```python
from build123d import *

# Parameters (mm, degrees)
SHELL1_T            = -1
LPATTERN1_COUNT     = 8
LPATTERN1_PITCH     = 9
SKETCH3_W           = 8
SKETCH3_H           = 92.26
BOSS_EXTRUDE1_DEPTH = 1
CHAMFER1_SIZE       = 1
SKETCH4_R           = 2.5
CUT_EXTRUDE1_DEPTH  = 82.991962069
CHAMFER2_SIZE       = 1
SKETCH5_W           = 3
SKETCH5_H           = 2
CUT_EXTRUDE2_DEPTH  = 84.346756649
LPATTERN2_COUNT     = 8
LPATTERN2_PITCH     = 9


with BuildPart() as part:
    # Sketch1 → Revolve1 (revolve)
    with BuildSketch(Plane.XY, mode=Mode.PRIVATE) as revolve1_sk:
        Polygon((0, 30), (3, 30), (3, 0), (2.1, -5), (0, -5), align=None)
    revolve(revolve1_sk.sketch.rotate(Axis((0, 30, 0), (0, -1, 0)), 180), axis=Axis((0, 30, 0), (0, -1, 0)))

    # Shell1
    shell1_openings = [part.faces().sort_by_distance(p)[0] for p in [
        (0, -5, 0),
        (0, 30, 0),
    ]]
    offset(amount=SHELL1_T, openings=shell1_openings, kind=Kind.INTERSECTION)


with BuildPart() as lpattern1_1:
    # LPattern1: pattern copy
    add(part.part.moved(Location(Vector(0, 0, 1) * (1 * LPATTERN1_PITCH))))


with BuildPart() as lpattern1_2:
    # LPattern1: pattern copy
    add(part.part.moved(Location(Vector(0, 0, 1) * (2 * LPATTERN1_PITCH))))


with BuildPart() as lpattern1_3:
    # LPattern1: pattern copy
    add(part.part.moved(Location(Vector(0, 0, 1) * (3 * LPATTERN1_PITCH))))


with BuildPart() as lpattern1_4:
    # LPattern1: pattern copy
    add(part.part.moved(Location(Vector(0, 0, 1) * (4 * LPATTERN1_PITCH))))


with BuildPart() as lpattern1_5:
    # LPattern1: pattern copy
    add(part.part.moved(Location(Vector(0, 0, 1) * (5 * LPATTERN1_PITCH))))


with BuildPart() as lpattern1_6:
    # LPattern1: pattern copy
    add(part.part.moved(Location(Vector(0, 0, 1) * (6 * LPATTERN1_PITCH))))


with BuildPart() as lpattern1_7:
    # LPattern1: pattern copy
    add(part.part.moved(Location(Vector(0, 0, 1) * (7 * LPATTERN1_PITCH))))


with BuildPart() as part_1:
    add(part.part)

    add(lpattern1_1.part)  # Boss-Extrude1 merges LPattern1_1

    add(lpattern1_2.part)  # Boss-Extrude1 merges LPattern1_2

    add(lpattern1_3.part)  # Boss-Extrude1 merges LPattern1_3

    add(lpattern1_4.part)  # Boss-Extrude1 merges LPattern1_4

    add(lpattern1_5.part)  # Boss-Extrude1 merges LPattern1_5

    add(lpattern1_6.part)  # Boss-Extrude1 merges LPattern1_6

    add(lpattern1_7.part)  # Boss-Extrude1 merges LPattern1_7
    # Sketch3 → Boss-Extrude1 (add, symmetric)
    with BuildSketch(Plane(origin=(0, 3, 0), x_dir=(-1, 0, 0), z_dir=(0, -1, 0))):
        with Locations((0, -31.527464831)):
            Rectangle(SKETCH3_W, SKETCH3_H)
    extrude(amount=BOSS_EXTRUDE1_DEPTH, both=True)

    # Chamfer1
    chamfer1_edges = [part_1.edges().sort_by_distance(p)[0] for p in [
        (3, 4, 0),
        (3, 2, 0),
        (3, 4, 9),
        (3, 2, 9),
        (3, 4, 18),
        (3, 2, 18),
        (3, 4, 27),
        (3, 2, 27),
        (3, 4, 36),
        (3, 2, 36),
        (3, 4, 45),
        (3, 2, 45),
        (3, 4, 54),
        (3, 2, 54),
        (3, 4, 63),
        (3, 2, 63),
    ]]
    chamfer(chamfer1_edges, length=CHAMFER1_SIZE - 0.0001)  # a hair under: the kernel refuses the full size

    # Sketch4 → Cut-Extrude1 (cut, through all)
    with BuildSketch(Plane(origin=(0, 4, 0), x_dir=(1, 0, 0), z_dir=(0, 1, 0))):
        with Locations(Location((0, -73.63, 0), (0, 0, 270))):
            Circle(SKETCH4_R)
        with Locations(Location((0, 10.63, 0), (0, 0, 270))):
            Circle(SKETCH4_R)
    extrude(amount=-CUT_EXTRUDE1_DEPTH, mode=Mode.SUBTRACT)

    # Chamfer2
    chamfer2_edges = [part_1.edges().sort_by_distance(p)[0] for p in [
        (0, 2, 71.13),
        (0, 4, 71.13),
        (0, 2, -13.13),
        (0, 4, -13.13),
    ]]
    chamfer(chamfer2_edges, length=CHAMFER2_SIZE - 0.0001)  # a hair under: the kernel refuses the full size

    # Sketch5 → Cut-Extrude2 (cut, symmetric)
    with BuildSketch(Plane(origin=(0, 0, 0), x_dir=(0, 0, -1), z_dir=(1, 0, 0))):
        with Locations((0, 29)):
            Rectangle(SKETCH5_W, SKETCH5_H)
    cut_extrude2 = extrude(amount=CUT_EXTRUDE2_DEPTH, both=True, mode=Mode.SUBTRACT)

    # LPattern2: Cut-Extrude2 ×8
    with Locations(*[(0, 0, i * LPATTERN2_PITCH) for i in range(1, LPATTERN2_COUNT)]):
        add(cut_extrude2, mode=Mode.SUBTRACT)


solid = part_1.part
```
Design review of the part built by this model. Coordinates are the model's own, in mm. A direction names the side the tool comes from. Coordinates: 2 decimals unless noted, no trailing zeros. Use CSV: the item, a comma, the result in double quotes. Start each with the question number.
1) The part is to be moulded in two halves that separate along X. For faces 5 (the cylindrical face through (-1.847, 16.818, 54.766)), 6 (the cylindrical face through (3, 17, 27)), 7 (the flat face through (-2.3, 28, 36)), say which applies: +X half, -X half, draft (parallel to the pull), parting line (faces both ways), or undercut.
2) Wall thickness on L1, parallel to X at y = 0.75, z = 54; L2, parallel to Y at x = -2.75, z = 57; L3, parallel to X at y = 3, z = 73: over which ranges is each line inside the solid? List them lowest first. Write a range as from..to.
3) For pin 1 Ø0.6 at (x, y) = (2, 29) entering from -Z; pin 2 Ø10 at (y, z) = (16.5, 39) entering from +X; pin 3 Ø0.8 at (x, z) = (2.5, 63) entering from +Y, all flat-tipped, find the tip position at first contact; note any pin that passes through.
4) Tool access review of faces 1 (the flat face through (2.4, 28, 9)), 2 (the conical face through (0.2, -2.491, 52.478)), 3 (the flat face through (0, 30, 24.7)), 4 (the flat face through (0, 4, 54)): name each direction out of +Z, -Z, +X, -X, +Y, -Y from which nothing blocks a thin tool from reaching the whole face with its end or side.
5) Consider section A-A on y = 22. Give the number of separate pieces and of enclosed holes in the cut face, then the cut area to 3 significant figures.
Geometry says:
1,face 5,"undercut"
1,face 6,"parting line"
1,face 7,"draft"
2,L1,"-3..-2, 2..3"
2,L2,"2..4"
2,L3,"-4..-2.42, 2.42..4"
3,pin 1,"z = -2.47"
3,pin 2,"x = 3"
3,pin 3,"y = 28"
4,face 1,"+X, -X, +Y"
4,face 2,"none"
4,face 3,"+Z, -Z, +X, -X, +Y"
4,face 4,"+Y"
5,separate pieces,"8"
5,enclosed holes,"8"
5,area,"126 mm^2"
